Model file for the job. Use its own axes, mm. Round coordinates to 2 decimals unless told otherwise and drop trailing zeros. Order: outer loops, then holes, each group sorted by start corner. A loop starts at its lowest first (then second) coordinate and runs counter-clockwise, first axis right, second up. Notation, with made-up numbers: (30, 73) - (74, 73) arc R10 cw to (74, 92) - close; hole circle Ø11 at (18, 71). An arc over 180 degrees is marked (long way). Use one line per item in the form item = value.
from build123d import *

# Parameters (mm, degrees)
SKETCH1_W           = 22
SKETCH1_H           = 16
BOSS_EXTRUDE1_DEPTH = 16
SKETCH2_R           = 4
CUT_EXTRUDE1_DEPTH  = 8
SKETCH3_R           = 4
CUT_EXTRUDE2_DEPTH  = 17


with BuildPart() as part:
    # Sketch1 → Boss-Extrude1 (new body)
    with BuildSketch(Plane.XY):
        with Locations((11, 8)):
            Rectangle(SKETCH1_W, SKETCH1_H)
    extrude(amount=BOSS_EXTRUDE1_DEPTH)

    # Sketch2 → Cut-Extrude1 (cut)
    with BuildSketch(Plane.ZY):
        with Locations(Location((8, 8, 0), (0, 0, 270))):  # turned: the seam where the file's is
            Circle(SKETCH2_R)
    extrude(amount=-CUT_EXTRUDE1_DEPTH, mode=Mode.SUBTRACT)

    # Sketch3 → Cut-Extrude2 (cut, through all)
    with BuildSketch(Plane.XZ):
        with Locations(Location((14, 8, 0), (0, 0, 270))):  # turned: the seam where the file's is
            Circle(SKETCH3_R)
    extrude(amount=-CUT_EXTRUDE2_DEPTH, mode=Mode.SUBTRACT)


solid = part.part
(1) Slice it at B-B on x = 14. Give the cut face in (y, z).
Report:
outline = (0, 0) - (16, 0) - (16, 4) - (0, 4) - close; (0, 12) - (16, 12) - (16, 16) - (0, 16) - close
(2) Slice it at C-C on y = 8. Give the cut face in (x, z), then the cut area to 3 significant figures.
Report:
outline = (0, 0) - (22, 0) - (22, 16) - (0, 16) - (0, 12) - (8, 12) - (8, 4) - (0, 4) - close; hole circle Ø8 at (14, 8)
area = 238 mm2
(3) Slice it at D-D on x = 2.75. Give the cut face in (y, z).
Report:
outline = (0, 0) - (16, 0) - (16, 16) - (0, 16) - close; hole circle Ø8 at (8, 8)
(4) Slice it at A-A on z = 8. Give the cut face in (x, y), then the cut area to 3 significant figures.
Report:
outline = (0, 0) - (10, 0) - (10, 16) - (0, 16) - (0, 12) - (8, 12) - (8, 4) - (0, 4) - close; (18, 0) - (22, 0) - (22, 16) - (18, 16) - close
area = 160 mm2
(5) Pull direction Y, two halves, no side cores. Call faces 1 (the face through (16.7, 7.89, 10.95)), 2 (the face through (8, 16, 8)), 3 (the face through (3.9, 11.2, 5.6)), 4 (the face through (8, 8, 8)): released by +Y, released by -Y, zero draft, split by the parting line, or undercut.
Report:
face_1 = zero draft
face_2 = released by +Y
face_3 = undercut
face_4 = undercut
(6) Pin check, flat tip, straight feed: pin 1 (5 mm diameter, centred on y = 8, z = 8, fed in from -X). Stop position of the tip, or through.
Report:
pin_1 = 8
(7) Probe probe 1 along X at (y, z) = (3.5, 8); probe 2 along Z at (x, y) = (5.5, 8); probe 3 along Z at (x, y) = (12.25, 7.25). List the from-to ranges inside material, lowest first. Write a range as [from, to].
Report:
probe_1 = [0, 10], [18, 22]
probe_2 = [0, 4], [12, 16]
probe_3 = [0, 4.4], [11.6, 16]
